Here's how the part is built. I have some questions about the finished solid (model axes, mm). Face numbers are marked on the shaded views. A direction names the side the tool comes from. Round coordinates to 2 decimals unless told otherwise and drop trailing zeros. Write each loop counter-clockwise with the first axis right and the second up, starting at its lowest first coordinate (ties: lowest second). Pieces come first, ordered by that corner, then holes. Notation, with made-up numbers: (12.5, -11.75) - (27.5, -11.75) arc R23 ccw to (27.5, 10.25) - close; hole circle Ø11 at (74, 87). An arc over 180 degrees is marked (long way). One line per item, written item: value. Start each with the question number.
Item 1: Imagine slicing it at A-A, the plane z = 0. Please give me the cut outline in (x, y) (1 decimal), then the cut area to 3 significant figures.
Item 2: For P1, Ø5, axis at y = 25, z = 8.5, coming from the -X side; P2, Ø4, axis at x = 0, z = 9.09, coming from the -Y side; P3, Ø8.5, axis at x = 0, z = 0, coming from the +Y side, each with a flat end and sliding along its axis, tell me the tip position at first contact or that it passes through.
Item 3: If I drill on line 1 (X direction, y = 1, z = 0) (1 decimal); line 2 (Y direction, x = 32.5, z = 4.5); line 3 (X direction, y = 30.5, z = -6) (3 decimals), over which ranges is the centre line in solid material (lowest first)?
Item 4: Imagine slicing it at C-C, the plane y = 44. Please give me the cut outline in (x, z) (1 decimal), then the cut area to 3 significant figures.
Item 5: Imagine slicing it at B-B, the plane x = 29. Please give me the cut outline in (y, z), then the cut area to 3 significant figures.
Item 6: For the marked faces 4 and 5, which set-ups out of +Z, -Z, +X, -X, +Y, -Y let a thin tool reach every point of the face, with its end or its side?
Item 7: Thinking about a two-plate mould opening in Y: for the marked faces 1, 2 and 3, which applies, released by +Y, released by -Y, zero draft, split by the parting line, or undercut?
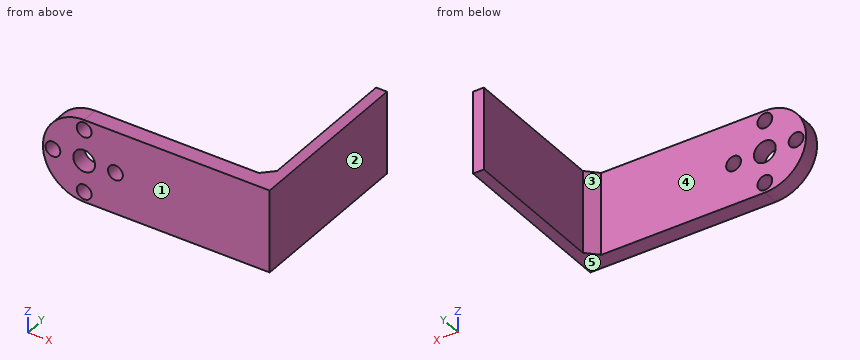
```python
from build123d import *

# Parameters (mm, degrees)
SKETCH1_R           = 2.159
SKETCH1_R_2         = 3.175
BOSS_EXTRUDE1_DEPTH = 4.7625
SKETCH1_3_W         = 3.175
SKETCH1_3_H         = 24.003
BOSS_EXTRUDE2_DEPTH = 50.8
CHAMFER1_SIZE       = 3.175


with BuildPart() as part:
    # Sketch1 → Boss-Extrude1 (new body)
    with BuildSketch(Plane(origin=(0, 0, 0), x_dir=(1, 0, 0), z_dir=(0, 1, 0))):
        with BuildLine():
            Line((50.8, 12.0015), (0, 12.0015))
            ThreePointArc((0, 12.0015), (-12.0015, 0), (0, -12.0015))
            Line((0, -12.0015), (50.8, -12.0015))
            Line((50.8, -12.0015), (50.8, 12.0015))
        make_face()
        with Locations(Location((-9.0932, 0, 0), (0, 0, 90))):
            Circle(SKETCH1_R, mode=Mode.SUBTRACT)
        with Locations(Location((0, -9.0932, 0), (0, 0, 90))):
            Circle(SKETCH1_R, mode=Mode.SUBTRACT)
        with Locations(Location((9.0932, 0, 0), (0, 0, 90))):
            Circle(SKETCH1_R, mode=Mode.SUBTRACT)
        with Locations(Location((0, 9.0932, 0), (0, 0, 90))):
            Circle(SKETCH1_R, mode=Mode.SUBTRACT)
        with Locations(Location((0, 0, 0), (0, 0, 90))):
            Circle(SKETCH1_R_2, mode=Mode.SUBTRACT)
    extrude(amount=BOSS_EXTRUDE1_DEPTH)

    # Sketch1_3 → Boss-Extrude2 (add)
    with BuildSketch(Plane(origin=(0, 0, 0), x_dir=(1, 0, 0), z_dir=(0, 1, 0))):
        with Locations((52.3875, 0)):
            Rectangle(SKETCH1_3_W, SKETCH1_3_H)
    extrude(amount=BOSS_EXTRUDE2_DEPTH)

    # Chamfer1
    chamfer1_edges = [part.edges().sort_by_distance(p)[0] for p in [
        (50.8, 4.7625, 0),
    ]]
    chamfer(chamfer1_edges, length=CHAMFER1_SIZE)


solid = part.part
```
Values follow:
1. outline: (-12, 0) - (-11.3, 0) - (-11.3, 4.8) - (-12, 4.8) - close; (-6.9, 0) - (-3.2, 0) - (-3.2, 4.8) - (-6.9, 4.8) - close; (3.2, 0) - (6.9, 0) - (6.9, 4.8) - (3.2, 4.8) - close; (11.3, 0) - (54, 0) - (54, 50.8) - (50.8, 50.8) - (50.8, 7.9) - (47.6, 4.8) - (11.3, 4.8) - close
1. area: 394 mm^2
2. P1: stops at x = 50.8
2. P2: passes through
2. P3: stops at y = 4.76
3. line 1: x = -12 to -11.3, -6.9 to -3.2, 3.2 to 6.9, 11.3 to 54
3. line 2: y = 0 to 4.76
3. line 3: x = 50.8 to 53.975
4. outline: (50.8, -12) - (54, -12) - (54, 12) - (50.8, 12) - close
4. area: 76.2 mm^2
5. outline: (0, -12) - (4.76, -12) - (4.76, 12) - (0, 12) - close
5. area: 114 mm^2
6. face 4: +Z, -Z, -X, +Y
6. face 5: -Z, +X, -X, +Y, -Y
7. face 1: released by -Y
7. face 2: zero draft
7. face 3: released by +Y
